from build123d import *

# Parameters (mm, degrees)
SKETCH1_W           = 150
SKETCH1_H           = 60
BOSS_EXTRUDE2_DEPTH = 60
SKETCH3_R           = 10
BOSS_EXTRUDE3_DEPTH = 5
SKETCH4_R           = 5
BOSS_EXTRUDE4_DEPTH = 5
SKETCH5_W           = 35
SKETCH5_H           = 10
BOSS_EXTRUDE5_DEPTH = 15
BOSS_EXTRUDE7_DEPTH = 10


with BuildPart() as part:
    # Sketch1 → Boss-Extrude2 (new body)
    with BuildSketch(Plane.XY):
        Rectangle(SKETCH1_W, SKETCH1_H)
    extrude(amount=-BOSS_EXTRUDE2_DEPTH)

    # Sketch3 → Boss-Extrude3 (add)
    with BuildSketch(Plane(origin=(0, 30, 0), x_dir=(1, 0, 0), z_dir=(0, 1, 0))):
        with Locations(Location((-60, 15, 0), (0, 0, 270))):
            Circle(SKETCH3_R)
    extrude(amount=BOSS_EXTRUDE3_DEPTH)

    # Sketch4 → Boss-Extrude4 (add)
    with BuildSketch(Plane(origin=(0, 35, 0), x_dir=(1, 0, 0), z_dir=(0, 1, 0))):
        with Locations(Location((-60, 15, 0), (0, 0, 270))):
            Circle(SKETCH4_R)
    extrude(amount=BOSS_EXTRUDE4_DEPTH)

    # Sketch5 → Boss-Extrude5 (add)
    with BuildSketch(Plane(origin=(75, 0, 0), x_dir=(0, 0, -1), z_dir=(1, 0, 0))):
        with Locations((30.361935687, 0.340382959)):
            Rectangle(SKETCH5_W, SKETCH5_H)
    extrude(amount=BOSS_EXTRUDE5_DEPTH)

    # Sketch6 → Boss-Extrude7 (add)
    with BuildSketch(Plane(origin=(0, 5.340382959, 0), x_dir=(1, 0, 0), z_dir=(0, 1, 0))):
        with BuildLine():
            Line((159.790141343, 1.592020078), (159.790141343, -11.203771863))
            ThreePointArc((159.790141343, -11.203771863), (82, 30.361935687), (159.790141343, 71.927643238))
            Line((159.790141343, 71.927643238), (159.790141343, 59.131851296))
            ThreePointArc((159.790141343, 59.131851296), (92, 30.361935687), (159.790141343, 1.592020078))
        make_face()
    extrude(amount=-BOSS_EXTRUDE7_DEPTH)


solid = part.part
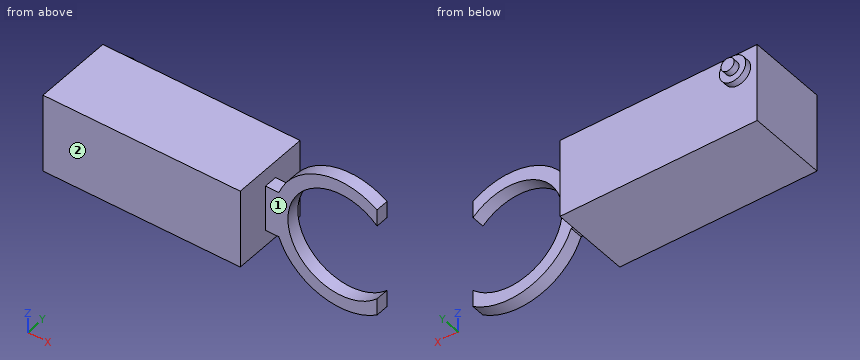
For this review, take the finished solid that the model builds, in its own axes (mm). Face numbers are marked on the shaded views. A direction names the side the tool comes from. Give positions to 0.01 mm unless a question says otherwise; leave off trailing zeros. Loops run counter-clockwise (first coordinate to the right, second up) from the corner with the lowest first, then second, coordinate; pieces in that order, holes last. Notation, with made-up numbers: (-22, 37) -> (12, 37) arc R12 cw to (12, 46) -> close; hole circle Ø3 at (-17, -5). An arc over 180 degrees is marked (long way). One line per question, with ' | ' between items.
1) We need section C-C (z = -15). Write out the cut boundary in (x, y).
Resolved:
outline: (-75, -30) -> (75, -30) -> (75, -4.66) -> (95.07, -4.66) -> (95.07, 5.34) -> (75, 5.34) -> (75, 30) -> (-50, 30) -> (-50, 35) -> (-55, 35) -> (-55, 40) -> (-65, 40) -> (-65, 35) -> (-70, 35) -> (-70, 30) -> (-75, 30) -> close
2) Insertion check: pin 1 Ø16 at (x, z) = (-63, -10) entering from +Y; pin 2 Ø3 at (x, y) = (-20, -14.5) entering from +Z; pin 3 Ø1.5 at (x, y) = (101.5, 3) entering from +Z; pin 4 Ø5 at (x, z) = (93, -53.5) entering from -Y. Each pin has a flat end and moves straight along its axis. Give the tip position at first contact, or say it passes through.
Resolved:
pin 1: stops at y = 40 | pin 2: stops at z = 0 | pin 3: stops at z = 9.82 | pin 4: stops at y = -4.66
3) To check wall thickness, follow probe 1 along Z at (x, y) = (132, 2.25); probe 2 along X at (y, z) = (-18, -1); probe 3 along Z at (x, y) = (51.5, -15). State the ranges of each line that lie inside material, in increasing order.
Resolved:
probe 1: z = -80.36 to -70.36, 9.64 to 19.64 | probe 2: x = -75 to 75 | probe 3: z = -60 to 0
4) We need section D-D (x = -60). Write out the cut boundary in (y, z).
Resolved:
outline: (-30, -60) -> (30, -60) -> (30, -25) -> (35, -25) -> (35, -20) -> (40, -20) -> (40, -10) -> (35, -10) -> (35, -5) -> (30, -5) -> (30, 0) -> (-30, 0) -> close
5) We need section A-A (z = -67). Write out the cut boundary in (x, y).
Resolved:
outline: (97.98, -4.66) -> (115.95, -4.66) -> (115.95, 5.34) -> (97.98, 5.34) -> close; (148.05, -4.66) -> (159.79, -4.66) -> (159.79, 5.34) -> (148.05, 5.34) -> close
6) For the marked faces 1 and 2, list the 3-axis set-ups (+Z, -Z, +X, -X, +Y, -Y) from which the entire face can be reached by the end or side of a thin tool; tool diameter is ignored.
Resolved:
face 1: +Z, -Z, +X, -Y | face 2: +Z, -Z, +X, -X, -Y
7) We need section B-B (x = 114). Write out the cut boundary in (y, z), plus the area to 3 significant figures.
Resolved:
outline: (-4.66, -77.01) -> (5.34, -77.01) -> (5.34, -66.08) -> (-4.66, -66.08) -> close; (-4.66, 5.36) -> (5.34, 5.36) -> (5.34, 16.29) -> (-4.66, 16.29) -> close | area: 219 mm2
